from build123d import *

# Parameters (mm, degrees)
DODANIE_WYCI_GNI_CIE1_DEPTH      = 9
DODANIE_WYCI_GNI_CIE1_DEPTH_BACK = 17
SZKIC1_R                         = 6.5
SZKIC1_R_2                       = 3
SZKIC1_3_R                       = 6.5
SZKIC1_3_R_2                     = 3
DODANIE_WYCI_GNI_CIE2_DEPTH      = 21
SFAZOWANIE1_SIZE                 = 2
SFAZOWANIE2_SIZE                 = 4
SZKIC3_R                         = 6
WYTNIJ_WYCI_GNI_CIE1_DEPTH       = 4
SFAZOWANIE3_SIZE                 = 1.5


with BuildPart() as part:
    # Szkic1 → Dodanie-wyci_gni_cie1 (new, two sides: drawn at the far end of the back side and taken through both)
    # profile 1 of 2: a face of its own
    with BuildSketch(Plane(origin=(0, 0, 0), x_dir=(1, 0, 0), z_dir=(0, 1, 0)).offset(-DODANIE_WYCI_GNI_CIE1_DEPTH_BACK)):
        Polygon((5.484827557, 9.5), (-5.484827557, 9.5), (-10.969655115, 0), (-5.484827557, -9.5), (5.484827557, -9.5), (10.969655115, 0), align=None)
        Circle(SZKIC1_R, mode=Mode.SUBTRACT)
    # profile 2 of 2: a face of its own
    with BuildSketch(Plane(origin=(0, 0, 0), x_dir=(1, 0, 0), z_dir=(0, 1, 0)).offset(-DODANIE_WYCI_GNI_CIE1_DEPTH_BACK)):
        Circle(SZKIC1_R)
        with Locations(Location((0, 0, 0), (0, 0, 270))):
            Circle(SZKIC1_R_2, mode=Mode.SUBTRACT)
    extrude(amount=DODANIE_WYCI_GNI_CIE1_DEPTH + DODANIE_WYCI_GNI_CIE1_DEPTH_BACK)

    # Szkic1_3 → Dodanie-wyci_gni_cie2 (add)
    with BuildSketch(Plane(origin=(0, 0, 0), x_dir=(1, 0, 0), z_dir=(0, 1, 0))):
        with Locations(Location((0, 0, 0), (0, 0, 90))):
            Circle(SZKIC1_3_R)
        with Locations(Location((0, 0, 0), (0, 0, 270))):
            Circle(SZKIC1_3_R_2, mode=Mode.SUBTRACT)
    extrude(amount=DODANIE_WYCI_GNI_CIE2_DEPTH)

    # Sfazowanie1
    sfazowanie1_edges = [part.edges().sort_by_distance(p)[0] for p in [
        (0, 21, -3),
    ]]
    chamfer(sfazowanie1_edges, length=SFAZOWANIE1_SIZE)

    # Sfazowanie2
    sfazowanie2_edges = [part.edges().sort_by_distance(p)[0] for p in [
        (0, -17, -3),
    ]]
    chamfer(sfazowanie2_edges, length=SFAZOWANIE2_SIZE)

    # Szkic3 → Wytnij-wyci_gni_cie1 (cut)
    with BuildSketch(Plane.XZ.offset(17)):
        with Locations(Location((0, 0, 0), (0, 0, 270))):
            Circle(SZKIC3_R)
    extrude(amount=-WYTNIJ_WYCI_GNI_CIE1_DEPTH, mode=Mode.SUBTRACT)

    # Sfazowanie3
    sfazowanie3_edges = [part.edges().sort_by_distance(p)[0] for p in [
        (0, -13, -3),
    ]]
    chamfer(sfazowanie3_edges, length=SFAZOWANIE3_SIZE)


solid = part.part
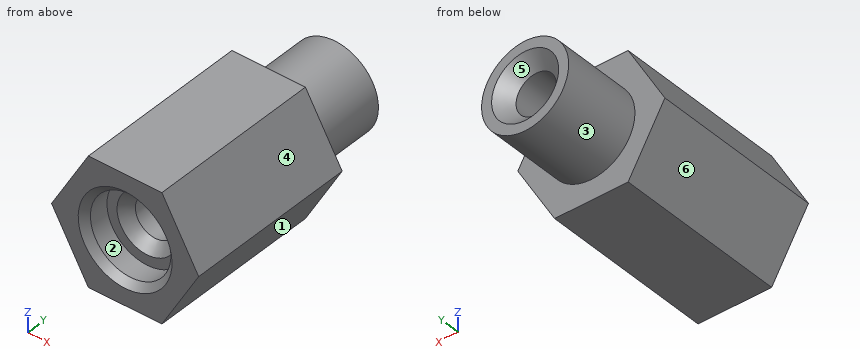
The listing builds one solid part. Answer for the finished solid, in the listing's coordinates (mm). Face numbers are marked on the shaded views. A direction names the side the tool comes from. Round coordinates to 2 decimals unless told otherwise and drop trailing zeros. Write each loop counter-clockwise with the first axis right and the second up, starting at its lowest first coordinate (ties: lowest second). Pieces come first, ordered by that corner, then holes. Notation, with made-up numbers: (86, 0) - (98, 0) arc R20 ccw to (98, 16) - close; hole circle Ø2 at (62, -8.5). An arc over 180 degrees is marked (long way). Use a Markdown table: item, result. Add a question column.
1. Flat-ended cylindrical pins translate along their axes: P1, Ø1.5, axis at x = 1, y = 10, coming from the -Z side; P2, Ø5, axis at y = 4, z = 5.5, coming from the +X side; P3, Ø11, axis at x = 0, z = 0, coming from the -Y side. Find the tip coordinate at first contact, or state that the pin passes through.
2. A tool of negligible diameter and unlimited length cuts with its end or side. For the marked faces 1, 2 and 3, from which of +Z, -Z, +X, -X, +Y, -Y can it reach the whole face along a straight path? Write none if from no direction.
3. The part is cut by section A-A (y = 8). Write down the section's boundary in (x, z), and give its area (3 significant figures).
4. The part is cut by section D-D (z = 7.5). Write down the section's boundary in (x, y).
5. The part is cut by section C-C (y = 16). Write down the section's boundary in (x, z).
6. For a pull along X with two mould halves and no side action, classify the marked faces 4, 5 and 6 as +X half, -X half, draft (parallel to the pull), parting line (faces both ways), or undercut.
7. The part is cut by section B-B (x = 0). Write down the section's boundary in (y, z), and give its area (3 significant figures).
8. Consider line 1 (X direction, y = 11.5, z = 0); line 2 (X direction, y = -14.4, z = 0); line 3 (Z direction, x = 0, y = -14.25). Determine where each line is inside the solid, lowest interval first.
Reported:
| question | item | result |
|---|---|---|
| 1 | P1 | z = -6.5 |
| 1 | P2 | x = 9.24 |
| 1 | P3 | y = -13 |
| 2 | face 1 | -Z, +X, +Y, -Y |
| 2 | face 2 | -Y |
| 2 | face 3 | +Y |
| 3 | outline | (-10.97, 0) - (-5.48, -9.5) - (5.48, -9.5) - (10.97, 0) - (5.48, 9.5) - (-5.48, 9.5) - close; hole circle Ø6 at (0, 0) |
| 3 | area | 284 mm^2 |
| 4 | outline | (-6.64, -17) - (6.64, -17) - (6.64, 9) - (-6.64, 9) - close |
| 5 | outline | circle Ø13 at (0, 0); hole circle Ø6 at (0, 0) |
| 6 | face 4 | +X half |
| 6 | face 5 | undercut |
| 6 | face 6 | -X half |
| 7 | outline | (-17, -9.5) - (9, -9.5) - (9, -6.5) - (21, -6.5) - (21, -5) - (19, -3) - (-11.5, -3) - (-13, -4.5) - (-13, -6) - (-16, -6) - (-17, -7) - close; (-17, 7) - (-16, 6) - (-13, 6) - (-13, 4.5) - (-11.5, 3) - (19, 3) - (21, 5) - (21, 6.5) - (9, 6.5) - (9, 9.5) - (-17, 9.5) - close |
| 7 | area | 391 mm^2 |
| 8 | line 1 | -6.5 to -3, 3 to 6.5 |
| 8 | line 2 | -10.97 to -6, 6 to 10.97 |
| 8 | line 3 | -9.5 to -6, 6 to 9.5 |
